Geometry: see drawing. Coordinates: mm, zero at the bounding-box minimum. A direction names the side the tool comes from. Coordinates: 2 decimals unless noted, no trailing zeros. Loops run counter-clockwise (first coordinate to the right, second up) from the corner with the lowest first, then second, coordinate; pieces in that order, holes last.
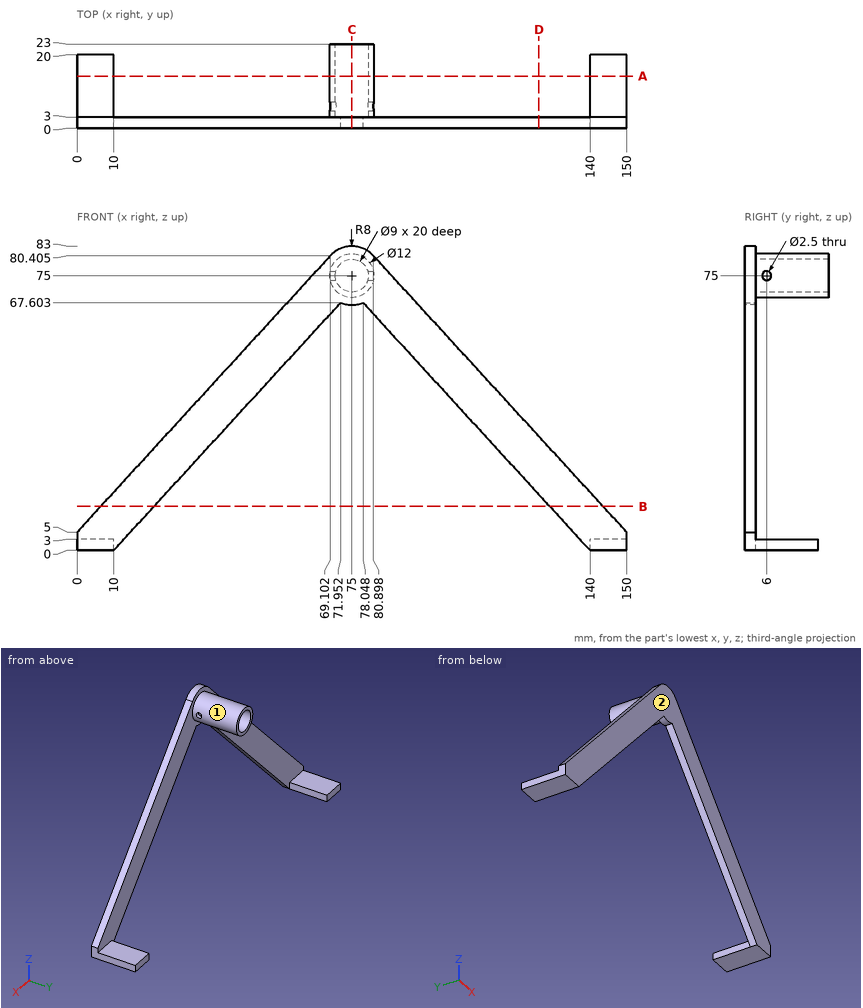
Item 1: Section query B-B (z = 12). Output: boundary loops of the cut face in (x, y) (1 decimal).
Result:
outline: (6.4, 0) - (21, 0) - (21, 3) - (6.4, 3) - close; (129, 0) - (143.6, 0) - (143.6, 3) - (129, 3) - close
Item 2: Line query: L1, parallel to Y at x = 70, z = 75; L2, parallel to Y at x = 36, z = 31; L3, parallel to X at y = 2.75, z = 25.5 (1 decimal). Output: solid intervals per line, ascending.
Result:
L1: y = 0 to 4.75, 7.25 to 23
L2: y = 0 to 3
L3: x = 18.8 to 33.4, 116.6 to 131.2
Item 3: Section query C-C (x = 75). Output: boundary loops of the cut face in (y, z), then the cut area to 3 significant figures.
Result:
outline: (0, 67) - (3, 67) - (3, 69) - (23, 69) - (23, 70.5) - (3, 70.5) - (3, 79.5) - (23, 79.5) - (23, 81) - (3, 81) - (3, 83) - (0, 83) - close
area: 108 mm2
Item 4: Section query D-D (x = 126). Output: boundary loops of the cut face in (y, z).
Result:
outline: (0, 15.28) - (3, 15.28) - (3, 31.19) - (0, 31.19) - close
Item 5: Contact query for flat-ended pins moving along their axis: P1, Ø3, axis at y = 6, z = 75, coming from the -X side; P2, Ø5, axis at x = 146, y = 14, coming from the +Z side; P3, Ø3.5, axis at x = 5, z = 2, coming from the +Y side. Output: stop coordinate, or through.
Result:
P1: stops at x = 69
P2: stops at z = 3
P3: stops at y = 20
Item 6: Section query A-A (y = 14.25). Output: boundary loops of the cut face in (x, z).
Result:
outline: (0, 0) - (10, 0) - (10, 3) - (0, 3) - close; circle Ø12 at (75, 75); (140, 0) - (150, 0) - (150, 3) - (140, 3) - close; hole circle Ø9 at (75, 75)
Item 7: Reachability of the marked faces 1 and 2 from +Z, -Z, +X, -X, +Y, -Y: full face, straight path, thin tool, end or side. Return the list, or none.
Result:
face 1: +Y
face 2: +Z, -Z, +X, -X, -Y
